```python
from build123d import *

# Parameters (mm, degrees)
BOSS_EXTRUDE1_DEPTH = 3
CUT_EXTRUDE1_REACH  = 5
SKETCH2_R           = 1.5
SKETCH6_W           = 3
SKETCH6_H           = 36
BOSS_EXTRUDE3_DEPTH = 8
SKETCH9_W           = 4
SKETCH9_H           = 6
BOSS_EXTRUDE4_DEPTH = 12
CUT_EXTRUDE2_REACH  = 6
SKETCH10_R          = 1
FILLET1_R           = 1.5


with BuildPart() as part:
    # Sketch1 → Boss-Extrude1 (new body)
    with BuildSketch(Plane.XY):
        Polygon((-18.5, 18), (18.5, 18), (18.5, 12), (7.5, 12), (7.5, -12), (18.5, -12), (18.5, -18), (-18.5, -18), align=None)
    extrude(amount=BOSS_EXTRUDE1_DEPTH)

    # Sketch2 → Cut-Extrude1 (cut, up to next)
    with BuildSketch(Plane.XY, mode=Mode.PRIVATE) as cut_extrude1_sk1:
        with Locations((-15, -14.5)):
            Circle(SKETCH2_R)
    cut_extrude1_tool1 = extrude(cut_extrude1_sk1.sketch, amount=CUT_EXTRUDE1_REACH, mode=Mode.PRIVATE) & part.part
    add(cut_extrude1_tool1.solids().sort_by_distance((-15, -14.5, 0))[0], mode=Mode.SUBTRACT)
    # Sketch2 → Cut-Extrude1 (cut, up to next)
    with BuildSketch(Plane.XY, mode=Mode.PRIVATE) as cut_extrude1_sk2:
        with Locations((15, -14.5)):
            Circle(SKETCH2_R)
    cut_extrude1_tool2 = extrude(cut_extrude1_sk2.sketch, amount=CUT_EXTRUDE1_REACH, mode=Mode.PRIVATE) & part.part
    add(cut_extrude1_tool2.solids().sort_by_distance((15, -14.5, 0))[0], mode=Mode.SUBTRACT)
    # Sketch2 → Cut-Extrude1 (cut, up to next)
    with BuildSketch(Plane.XY, mode=Mode.PRIVATE) as cut_extrude1_sk3:
        with Locations((15, 14.5)):
            Circle(SKETCH2_R)
    cut_extrude1_tool3 = extrude(cut_extrude1_sk3.sketch, amount=CUT_EXTRUDE1_REACH, mode=Mode.PRIVATE) & part.part
    add(cut_extrude1_tool3.solids().sort_by_distance((15, 14.5, 0))[0], mode=Mode.SUBTRACT)
    # Sketch2 → Cut-Extrude1 (cut, up to next)
    with BuildSketch(Plane.XY, mode=Mode.PRIVATE) as cut_extrude1_sk4:
        with Locations((-15, 14.5)):
            Circle(SKETCH2_R)
    cut_extrude1_tool4 = extrude(cut_extrude1_sk4.sketch, amount=CUT_EXTRUDE1_REACH, mode=Mode.PRIVATE) & part.part
    add(cut_extrude1_tool4.solids().sort_by_distance((-15, 14.5, 0))[0], mode=Mode.SUBTRACT)

    # Sketch6 → Boss-Extrude3 (add)
    with BuildSketch(Plane.ZY.offset(18.5)):
        with Locations((1.5, 0)):
            Rectangle(SKETCH6_W, SKETCH6_H)
    extrude(amount=BOSS_EXTRUDE3_DEPTH)

    # Sketch9 → Boss-Extrude4 (add)
    with BuildSketch(Plane.XY):
        with Locations((-24.5, 15)):
            Rectangle(SKETCH9_W, SKETCH9_H)
        with Locations((-24.5, -15)):
            Rectangle(SKETCH9_W, SKETCH9_H)
    extrude(amount=-BOSS_EXTRUDE4_DEPTH)

    # Sketch10 → Cut-Extrude2 (cut, up to next)
    with BuildSketch(Plane(origin=(-22.5, 0, 0), x_dir=(0, 0, -1), z_dir=(1, 0, 0)), mode=Mode.PRIVATE) as cut_extrude2_sk1:
        with Locations((6, 14)):
            Circle(SKETCH10_R)
    cut_extrude2_tool1 = extrude(cut_extrude2_sk1.sketch, amount=-CUT_EXTRUDE2_REACH, mode=Mode.PRIVATE) & part.part
    add(cut_extrude2_tool1.solids().sort_by_distance((-22.5, 14, -6))[0], mode=Mode.SUBTRACT)
    # Sketch10 → Cut-Extrude2 (cut, up to next)
    with BuildSketch(Plane(origin=(-22.5, 0, 0), x_dir=(0, 0, -1), z_dir=(1, 0, 0)), mode=Mode.PRIVATE) as cut_extrude2_sk2:
        with Locations((6, -14)):
            Circle(SKETCH10_R)
    cut_extrude2_tool2 = extrude(cut_extrude2_sk2.sketch, amount=-CUT_EXTRUDE2_REACH, mode=Mode.PRIVATE) & part.part
    add(cut_extrude2_tool2.solids().sort_by_distance((-22.5, -14, -6))[0], mode=Mode.SUBTRACT)

    # Fillet1
    fillet1_edges = [part.edges().sort_by_distance(p)[0] for p in [
        (-24.5, 12, 0),
        (-22.5, 15, 0),
        (-24.5, -12, 0),
        (-22.5, -15, 0),
    ]]
    fillet(fillet1_edges, radius=FILLET1_R)


solid = part.part
```
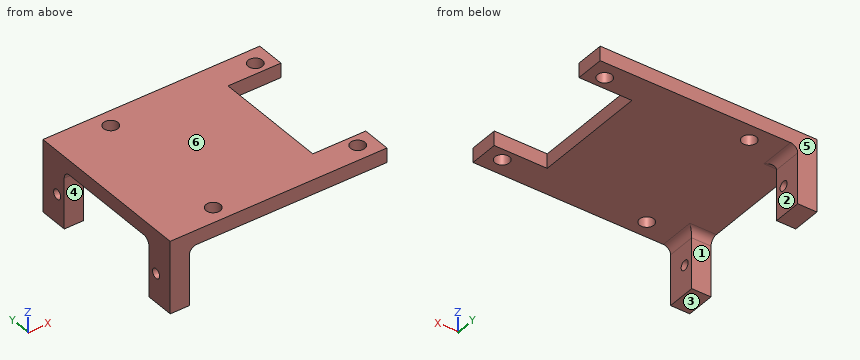
Read the model definition and answer for the solid it produces. Units are mm, in the model's axes. Face numbers are marked on the shaded views. A direction names the side the tool comes from. Give positions to 0.01 mm unless a question says otherwise; leave off trailing zeros. Order: outer loops, then holes, each group sorted by start corner. A loop starts at its lowest first (then second) coordinate and runs counter-clockwise, first axis right, second up.
(1) Given pin 1 (6.5 mm diameter, centred on y = -16.5, z = -5.5, fed in from +X); pin 2 (1.5 mm diameter, centred on y = 1, z = 1.5, fed in from +X); pin 3 (11 mm diameter, centred on x = -7.5, y = -2.5, fed in from -Z), each flat-ended and moving along its own axis, determine where each tip first touches the part or whether it passes through.
(2) Straight lines are drawn through the part: L1, parallel to Y at x = -15, z = 1.25; L2, parallel to Y at x = -24.1, z = -6; L3, parallel to Y at x = 15, z = 0.85. For each, find the intervals that lie inside material, in ascending order.
(3) Find section D-D (z = -6). Give the vertices of the cut face in (x, y), plus the area to 3 significant figures.
(4) For the marked faces 1, 2 and 3, determine the directions among +Z, -Z, +X, -X, +Y, -Y from which every point of the face is accessible in a straight line to the end or side of a thin tool.
(5) Find section A-A (x = 15). Give the vertices of the cut face in (y, z).
(6) Find section B-B (z = -10.5). Give the vertices of the cut face in (x, y), plus the area to 3 significant figures.
(7) Find section C-C (x = -15). Give the vertices of the cut face in (y, z), plus the area to 3 significant figures.
(8) For a pull along Y with two mould halves and no side action, classify the marked faces 4, 5 and 6 as released by +Y, released by -Y, zero draft, split by the parting line, or undercut.
Result sheet:
1. pin 1: stops at x = -22.5
1. pin 2: stops at x = 7.5
1. pin 3: stops at z = 0
2. L1: y = -18 to -16, -13 to 13, 16 to 18
2. L2: y = -18 to -15, -13 to -12, 12 to 13, 15 to 18
2. L3: y = -18 to -16, -13 to -12, 12 to 13, 16 to 18
3. outline: (-26.5, -18) - (-22.5, -18) - (-22.5, -15) - (-26.5, -15) - close; (-26.5, -13) - (-22.5, -13) - (-22.5, -12) - (-26.5, -12) - close; (-26.5, 12) - (-22.5, 12) - (-22.5, 13) - (-26.5, 13) - close; (-26.5, 15) - (-22.5, 15) - (-22.5, 18) - (-26.5, 18) - close
3. area: 32.0 mm2
4. face 1: -Z, +X, -X
4. face 2: -Z, +X, +Y, -Y
4. face 3: -Z, +X, -X, +Y, -Y
5. outline: (-18, 0) - (-16, 0) - (-16, 3) - (-18, 3) - close; (-13, 0) - (-12, 0) - (-12, 3) - (-13, 3) - close; (12, 0) - (13, 0) - (13, 3) - (12, 3) - close; (16, 0) - (18, 0) - (18, 3) - (16, 3) - close
6. outline: (-26.5, -18) - (-22.5, -18) - (-22.5, -12) - (-26.5, -12) - close; (-26.5, 12) - (-22.5, 12) - (-22.5, 18) - (-26.5, 18) - close
6. area: 48.0 mm2
7. outline: (-18, 0) - (-16, 0) - (-16, 3) - (-18, 3) - close; (-13, 0) - (13, 0) - (13, 3) - (-13, 3) - close; (16, 0) - (18, 0) - (18, 3) - (16, 3) - close
7. area: 90.0 mm2
8. face 4: undercut
8. face 5: released by +Y
8. face 6: zero draft
